Input: part model. Units: mm. Frame: model coordinates. A direction names the side the tool comes from. Coordinates: 2 decimals unless noted, no trailing zeros. Write each loop counter-clockwise with the first axis right and the second up, starting at its lowest first coordinate (ties: lowest second). Pieces come first, ordered by that corner, then holes. Notation, with made-up numbers: M 0.5,50.5 L 5.5,50.5 A16 cw 5.5,62.5 Z; hole C 31,15 d7. An arc over 180 degrees is marked long. Use CSV: the item, a comma, the result in double quotes.
```python
from build123d import *

# Parameters (mm, degrees)
SKETCH1_R           = 2.4892
BOSS_EXTRUDE1_DEPTH = 3.175
CUT_EXTRUDE1_DEPTH  = 113.028470154
FILLET1_R           = 5.08


with BuildPart() as part:
    # Sketch1 → Boss-Extrude1 (new, symmetric)
    with BuildSketch(Plane.XY):
        Polygon((-57.15, 92.075), (57.15, 92.075), (63.5, 50.8), (63.5, 0), (-63.5, 0), (-63.5, 50.8), align=None)
        with Locations((44.45, 73.025)):
            Circle(SKETCH1_R, mode=Mode.SUBTRACT)
        with Locations((44.45, 85.725)):
            Circle(SKETCH1_R, mode=Mode.SUBTRACT)
        with Locations(Location((-44.45, 73.025, 0), (0, 0, 180))):
            Circle(SKETCH1_R, mode=Mode.SUBTRACT)
        with Locations(Location((-44.45, 85.725, 0), (0, 0, 180))):
            Circle(SKETCH1_R, mode=Mode.SUBTRACT)
        with Locations((6.35, 12.7)):
            Circle(SKETCH1_R, mode=Mode.SUBTRACT)
        with Locations((6.35, 25.4)):
            Circle(SKETCH1_R, mode=Mode.SUBTRACT)
        with Locations((6.35, 38.1)):
            Circle(SKETCH1_R, mode=Mode.SUBTRACT)
        with Locations((19.05, 38.1)):
            Circle(SKETCH1_R, mode=Mode.SUBTRACT)
        with Locations((19.05, 25.4)):
            Circle(SKETCH1_R, mode=Mode.SUBTRACT)
        with Locations((19.05, 12.7)):
            Circle(SKETCH1_R, mode=Mode.SUBTRACT)
        with Locations((31.75, 38.1)):
            Circle(SKETCH1_R, mode=Mode.SUBTRACT)
        with Locations((31.75, 25.4)):
            Circle(SKETCH1_R, mode=Mode.SUBTRACT)
        with Locations((31.75, 12.7)):
            Circle(SKETCH1_R, mode=Mode.SUBTRACT)
        with Locations((44.45, 38.1)):
            Circle(SKETCH1_R, mode=Mode.SUBTRACT)
        with Locations((44.45, 25.4)):
            Circle(SKETCH1_R, mode=Mode.SUBTRACT)
        with Locations((44.45, 12.7)):
            Circle(SKETCH1_R, mode=Mode.SUBTRACT)
        with Locations((-6.35, 12.7)):
            Circle(SKETCH1_R, mode=Mode.SUBTRACT)
        with Locations((-6.35, 25.4)):
            Circle(SKETCH1_R, mode=Mode.SUBTRACT)
        with Locations((-6.35, 38.1)):
            Circle(SKETCH1_R, mode=Mode.SUBTRACT)
        with Locations((-19.05, 12.7)):
            Circle(SKETCH1_R, mode=Mode.SUBTRACT)
        with Locations((-19.05, 25.4)):
            Circle(SKETCH1_R, mode=Mode.SUBTRACT)
        with Locations((-19.05, 38.1)):
            Circle(SKETCH1_R, mode=Mode.SUBTRACT)
        with Locations((-31.75, 12.7)):
            Circle(SKETCH1_R, mode=Mode.SUBTRACT)
        with Locations((-31.75, 25.4)):
            Circle(SKETCH1_R, mode=Mode.SUBTRACT)
        with Locations((-31.75, 38.1)):
            Circle(SKETCH1_R, mode=Mode.SUBTRACT)
        with Locations((-44.45, 12.7)):
            Circle(SKETCH1_R, mode=Mode.SUBTRACT)
        with Locations((-44.45, 25.4)):
            Circle(SKETCH1_R, mode=Mode.SUBTRACT)
        with Locations((-44.45, 38.1)):
            Circle(SKETCH1_R, mode=Mode.SUBTRACT)
        with Locations((57.15, 38.1)):
            Circle(SKETCH1_R, mode=Mode.SUBTRACT)
        with Locations((57.15, 25.4)):
            Circle(SKETCH1_R, mode=Mode.SUBTRACT)
        with Locations((57.15, 12.7)):
            Circle(SKETCH1_R, mode=Mode.SUBTRACT)
        with Locations((-57.15, 12.7)):
            Circle(SKETCH1_R, mode=Mode.SUBTRACT)
        with Locations((-57.15, 25.4)):
            Circle(SKETCH1_R, mode=Mode.SUBTRACT)
        with Locations((-57.15, 38.1)):
            Circle(SKETCH1_R, mode=Mode.SUBTRACT)
    extrude(amount=BOSS_EXTRUDE1_DEPTH, both=True)

    # Sketch2 → Cut-Extrude1 (cut, through all)
    with BuildSketch(Plane.XY.offset(3.175)):
        Polygon((-38.1, 79.375), (-6.35, 79.375), (-6.35, 46.0375), (-51.383275403, 46.0375), (-48.208275403, 66.675), (-38.1, 66.675), align=None)
        Polygon((38.1, 79.375), (38.1, 66.675), (48.208275403, 66.675), (51.383275403, 46.0375), (6.35, 46.0375), (6.35, 79.375), align=None)
    extrude(amount=-CUT_EXTRUDE1_DEPTH, mode=Mode.SUBTRACT)

    # Fillet1
    fillet1_edges = [part.edges().sort_by_distance(p)[0] for p in [
        (-57.15, 92.075, 0),
        (57.15, 92.075, 0),
        (63.5, 50.8, 0),
        (63.5, 0, 0),
        (-63.5, 0, 0),
        (-63.5, 50.8, 0),
        (-6.35, 79.375, 0),
        (-6.35, 46.0375, 0),
        (-51.383275403, 46.0375, 0),
        (-48.208275403, 66.675, 0),
        (-38.1, 66.675, 0),
        (-38.1, 79.375, 0),
        (6.35, 79.375, 0),
        (38.1, 79.375, 0),
        (38.1, 66.675, 0),
        (48.208275403, 66.675, 0),
        (51.383275403, 46.0375, 0),
        (6.35, 46.0375, 0),
    ]]
    fillet(fillet1_edges, radius=FILLET1_R)


solid = part.part
```
1. Mould query, pull axis X, two halves, no side actions, for faces 1 (the cylindrical face through (-62.051, 1.528, 0.044)), 2 (the cylindrical face through (62.051, 1.528, -0.044)), 3 (the flat face through (38.1, 73, 0)). Classes: pulls with the +X half, pulls with the -X half, needs draft (parallel to the pull), parting line crosses it, or undercut.
Resolved:
face 1,"pulls with the -X half"
face 2,"pulls with the +X half"
face 3,"undercut"
2. Section C-C (y = 61). Return loops of the section in (x, z) (3 decimals), then the cut area to 3 significant figures.
Resolved:
outline,"M -61.931,-3.175 L -49.081,-3.175 L -49.081,3.175 L -61.931,3.175 Z; M -6.35,-3.175 L 6.35,-3.175 L 6.35,3.175 L -6.35,3.175 Z; M 49.081,-3.175 L 61.931,-3.175 L 61.931,3.175 L 49.081,3.175 Z"
area,"244 mm^2"
3. Section A-A (x = 26.5). Return loops of the section in (y, z) (1 decimal), then the cut area to 3 significant figures.
Resolved:
outline,"M 0,-3.2 L 46,-3.2 L 46,3.2 L 0,3.2 Z; M 79.4,-3.2 L 92.1,-3.2 L 92.1,3.2 L 79.4,3.2 Z"
area,"373 mm^2"
4. Section B-B (x = -19.05). Return loops of the section in (y, z) (1 decimal), then the cut area to 3 significant figures.
Resolved:
outline,"M 0,-3.2 L 10.2,-3.2 L 10.2,3.2 L 0,3.2 Z; M 15.2,-3.2 L 22.9,-3.2 L 22.9,3.2 L 15.2,3.2 Z; M 27.9,-3.2 L 35.6,-3.2 L 35.6,3.2 L 27.9,3.2 Z; M 40.6,-3.2 L 46,-3.2 L 46,3.2 L 40.6,3.2 Z; M 79.4,-3.2 L 92.1,-3.2 L 92.1,3.2 L 79.4,3.2 Z"
area,"278 mm^2"
5. Contact query for flat-ended pins moving along their axis: pin 1 Ø8 at (x, y) = (-31.75, 25.4) entering from -Z (3 decimals); pin 2 Ø2 at (y, z) = (73.5, 1) entering from +X. Output: stop coordinate, or through.
Resolved:
pin 1,"stops at z = -3.175"
pin 2,"stops at x = 60.16"
6. Section D-D (y = 12.7). State how many separate pieces and enclosed holes the cut face has, then the cut area to 3 significant figures.
Resolved:
separate pieces,"11"
enclosed holes,"0"
area,"490 mm^2"
7. Material intervals for line 1 (Y direction, x = -19.05, z = -1) (1 decimal); line 2 (X direction, y = 70, z = -2); line 3 (Y direction, x = -25.5, z = -3) (1 decimal), sorted ascending. Write a range as [from, to].
Resolved:
line 1,"y = [0, 10.2], [15.2, 22.9], [27.9, 35.6], [40.6, 46], [79.4, 92.1]"
line 2,"x = [-60.55, -38.41], [-6.35, 6.35], [38.41, 60.55]"
line 3,"y = [0, 46], [79.4, 92.1]"
8. Access query for faces 4 (the flat face through (-22, 79.375, 0)), 5 (the cylindrical face through (-56.061, 90.883, 0.044)). Directions: +Z, -Z, +X, -X, +Y, -Y. A direction counts if a zero-diameter tool reaches every point of the face in a straight line with its end or side. Return the directions, or none.
Resolved:
face 4,"+Z, -Z"
face 5,"+Z, -Z, -X, +Y"
